Part model, mm, in its own coordinate system. A direction names the side the tool comes from. Coordinates: 2 decimals unless noted, no trailing zeros. Loops run counter-clockwise (first coordinate to the right, second up) from the corner with the lowest first, then second, coordinate; pieces in that order, holes last. Notation, with made-up numbers: (49, 68) - (83, 68) arc R25 ccw to (83, 86) - close; hole circle Ø2 at (-35.75, 64.25). An arc over 180 degrees is marked (long way). Use a Markdown table: item, result. Add a question column.
1) Band-saw the part on B-B (y = 0). Give the cut face in (x, z).
2) Drop flat-ended pins along their axis: P1, Ø8, axis at x = 0, y = 0, coming from the +Z side; P2, Ø2.5, axis at x = 0.5, y = -0.5, coming from the -Z side. Give the stop position or say it passes through.
3) Tool access for faces 4 (the face through (4.5, -7.4, 1)), 5 (the face through (6.445, -2.945, 0.944)), 6 (the face through (-1, 1, -1)): list every direction of +Z, -Z, +X, -X, +Y, -Y with a clear straight run to the whole face (end or side of a thin tool).
4) Probe probe 1 along Y at (x, z) = (0, 2.5); probe 2 along Y at (x, z) = (0, -2.5); probe 3 along X at (y, z) = (2.5, 1.5). List the from-to ranges inside material, lowest first. Write a range as [from, to].
5) Band-saw the part on A-A (z = -0.5). Give the cut face in (x, y).
6) Pull direction X, two halves, no side cores. Call faces 1 (the face through (-4.27, -2.16, 0.94)), 2 (the face through (4.57, 7.167, 2.972)), 3 (the face through (0, -2, 5)): +X half, -X half, draft (parallel to the pull), parting line (faces both ways), or undercut.
7) Band-saw the part on C-C (x = 0). Give the cut face in (y, z).
8) Band-saw the part on D-D (y = 3). Give the cut face in (x, z), plus the area to 3 significant figures.
from build123d import *
from build123d.topology import SkipClean

# Parameters (mm, degrees)
SKETCH_1_R          = 8.5
SKETCH_1_R_2        = 2.5
EXTRUDE_1_DEPTH     = 5
SKETCH_2_R          = 1.25
CUT_EXTRUDE_1_DEPTH = 5
SKETCH_3_R          = 10
SKETCH_3_R_2        = 8.5
EXTRUDE_2_DEPTH     = 1
EXTRUDE_START       = 3
SKETCH_4_R          = 10
SKETCH_4_R_2        = 2.5
SKETCH_4_R_3        = 1.25
EXTRUDE_3_DEPTH     = 3
EXTRUDE_START_2     = -6
SKETCH_5_R          = 2.5
EXTRUDE_4_DEPTH     = 6
SKETCH_7_R          = 1
CUT_EXTRUDE_2_DEPTH = 10


with BuildPart() as part:
    # 草图1 → 凸台-拉伸1 (new body)
    with BuildSketch(Plane.XY):
        Circle(SKETCH_1_R)
        Circle(SKETCH_1_R_2, mode=Mode.SUBTRACT)
    extrude(amount=EXTRUDE_1_DEPTH)

    # 草图2 → 切除-拉伸1 (cut)
    with BuildSketch(Plane(origin=(0, 0, 0), x_dir=(-1, 0, 0), z_dir=(0, 0, -1))):
        with Locations((0, 6)):
            Circle(SKETCH_2_R)
        with Locations((5.196152423, 3)):
            Circle(SKETCH_2_R)
        with Locations((5.196152423, -3)):
            Circle(SKETCH_2_R)
        with Locations((0, -6)):
            Circle(SKETCH_2_R)
        with Locations((-5.196152423, -3)):
            Circle(SKETCH_2_R)
        with Locations((-5.196152423, 3)):
            Circle(SKETCH_2_R)
    extrude(amount=-CUT_EXTRUDE_1_DEPTH, mode=Mode.SUBTRACT)

    # 草图3 → 凸台-拉伸2 (add)
    with BuildSketch(Plane(origin=(0, 0, 0), x_dir=(-1, 0, 0), z_dir=(0, 0, -1))):
        Circle(SKETCH_3_R)
        Circle(SKETCH_3_R_2, mode=Mode.SUBTRACT)
    extrude(amount=-EXTRUDE_2_DEPTH)

    # 草图4 → 凸台-拉伸3 (add)
    with SkipClean():  # the faces are left unmerged after this step: merging them gives an invalid solid
        with BuildSketch(Plane(origin=(0, 0, 0), x_dir=(-1, 0, 0), z_dir=(0, 0, -1)).offset(EXTRUDE_START)):
            Circle(SKETCH_4_R)
            Circle(SKETCH_4_R_2, mode=Mode.SUBTRACT)
            with Locations((0, 6)):
                Circle(SKETCH_4_R_3, mode=Mode.SUBTRACT)
            with Locations((5.196152423, 3)):
                Circle(SKETCH_4_R_3, mode=Mode.SUBTRACT)
            with Locations((5.196152423, -3)):
                Circle(SKETCH_4_R_3, mode=Mode.SUBTRACT)
            with Locations((0, -6)):
                Circle(SKETCH_4_R_3, mode=Mode.SUBTRACT)
            with Locations((-5.196152423, -3)):
                Circle(SKETCH_4_R_3, mode=Mode.SUBTRACT)
            with Locations((-5.196152423, 3)):
                Circle(SKETCH_4_R_3, mode=Mode.SUBTRACT)
        extrude(amount=-EXTRUDE_3_DEPTH)

    # 草图5 → 凸台-拉伸4 (add)
    with BuildSketch(Plane.XY.offset(5).offset(EXTRUDE_START_2)):
        with Locations(Location((0, 0, 0), (0, 0, 180))):
            Circle(SKETCH_5_R)
    extrude(amount=EXTRUDE_4_DEPTH)

    # 草图7 → 切除-拉伸2 (cut)
    with BuildSketch(Plane(origin=(0, 0, -1), x_dir=(-1, 0, 0), z_dir=(0, 0, -1))):
        Circle(SKETCH_7_R)
    extrude(amount=-CUT_EXTRUDE_2_DEPTH, mode=Mode.SUBTRACT)


solid = part.part
Answer block:
| question | item | result |
|---|---|---|
| 1 | outline | (-10, -3) - (-2.5, -3) - (-2.5, -1) - (-1, -1) - (-1, 5) - (-8.5, 5) - (-8.5, 1) - (-10, 1) - close; (1, -1) - (2.5, -1) - (2.5, -3) - (10, -3) - (10, 1) - (8.5, 1) - (8.5, 5) - (1, 5) - close |
| 2 | P1 | z = 5 |
| 2 | P2 | z = -1 |
| 3 | face 4 | +Z |
| 3 | face 5 | +Z, -Z |
| 3 | face 6 | -Z |
| 4 | probe 1 | [-8.5, -7.25], [-4.75, -1], [1, 4.75], [7.25, 8.5] |
| 4 | probe 2 | [-10, -7.25], [-4.75, -2.5], [2.5, 4.75], [7.25, 10] |
| 4 | probe 3 | [-8.12, -6.34], [-4.05, 4.05], [6.34, 8.12] |
| 5 | outline | circle Ø20 at (0, 0); hole circle Ø2.5 at (-5.2, -3); hole circle Ø2.5 at (-5.2, 3); hole circle Ø2.5 at (0, -6); hole circle Ø2.5 at (0, 6); hole circle Ø2 at (0, 0); hole circle Ø2.5 at (5.2, -3); hole circle Ø2.5 at (5.2, 3) |
| 6 | face 1 | undercut |
| 6 | face 2 | parting line |
| 6 | face 3 | draft |
| 7 | outline | (-10, -3) - (-7.25, -3) - (-7.25, 5) - (-8.5, 5) - (-8.5, 1) - (-10, 1) - close; (-4.75, -3) - (-2.5, -3) - (-2.5, -1) - (-1, -1) - (-1, 5) - (-4.75, 5) - close; (1, -1) - (2.5, -1) - (2.5, -3) - (4.75, -3) - (4.75, 5) - (1, 5) - close; (7.25, -3) - (10, -3) - (10, 1) - (8.5, 1) - (8.5, 5) - (7.25, 5) - close |
| 8 | outline | (-9.54, -3) - (-6.45, -3) - (-6.45, 5) - (-7.95, 5) - (-7.95, 1) - (-9.54, 1) - close; (-3.95, -3) - (3.95, -3) - (3.95, 5) - (-3.95, 5) - close; (6.45, -3) - (9.54, -3) - (9.54, 1) - (7.95, 1) - (7.95, 5) - (6.45, 5) - close |
| 8 | area | 99.9 mm2 |
